```python
from build123d import *

# Parameters (mm, degrees)
HOLE1_D           = 16.0147
HOLE1_DEPTH       = 58.7248
HOLE1_CSINK_D     = 17.5387
HOLE1_CSINK_ANGLE = 90


with BuildPart() as part:
    # Sketch1 → Revolve1 (revolve)
    with BuildSketch(Plane.XY):
        with BuildLine():
            Line((0, 0), (0, 14.61516))
            Line((0, 14.61516), (1.25984, 15.875))
            Line((1.25984, 15.875), (12.006992339, 15.875))
            Line((12.006992339, 15.875), (13.283429147, 14.641164804))
            ThreePointArc((13.283429147, 14.641164804), (13.72258185, 14.355749006), (14.2367, 14.25575))
            Line((14.2367, 14.25575), (16.1036, 14.25575))
            ThreePointArc((16.1036, 14.25575), (17.073467661, 14.657482339), (17.4752, 15.62735))
            Line((17.4752, 15.62735), (17.4752, 17.44345))
            Line((17.4752, 17.44345), (20.6502, 17.44345))
            Line((20.6502, 17.44345), (20.6502, 0))
            Line((20.6502, 0), (0, 0))
        make_face()
    revolve(axis=Axis((20.6502, 0, 0), (-1, 0, 0)))

    # Sketch2 → Revolve2 (revolve)
    with BuildSketch(Plane.XY):
        Polygon((20.6502, 0), (20.6502, 24.96185), (22.1742, 26.48585), (49.1998, 26.48585), (49.1998, 24.51735), (50.2539, 24.51735), (51.308, 25.57145), (57.9628, 25.57145), (58.7248, 24.80945), (58.7248, 0), align=None)
    revolve(axis=Axis((58.7248, 0, 0), (-1, 0, 0)))

    # Hole1
    with Locations(Plane.ZY):
        with Locations((0, 0)):
            CounterSinkHole(HOLE1_D / 2, HOLE1_CSINK_D / 2, depth=HOLE1_DEPTH, counter_sink_angle=HOLE1_CSINK_ANGLE)

    # Sketch5 → Cut-Revolve1 (revolve, cut)
    with BuildSketch(Plane(origin=(0, 0, 0), x_dir=(1, 0, 0), z_dir=(0, 1, 0))):
        Polygon((39.1668, 0), (42.3418, 0), (42.3418, -8.986753545), (45.108896455, -11.75385), (45.568822746, -26.48585), (39.1668, -26.48585), align=None)
    revolve(axis=Axis((39.1668, 0, 26.48585), (0, 0, -1)), mode=Mode.SUBTRACT)

    # Sketch6 → Revolve3 (revolve)
    with BuildSketch(Plane.XY):
        with BuildLine():
            Line((49.1998, 24.26335), (50.2539, 24.26335))
            Line((50.2539, 24.26335), (50.2539, 24.51735))
            Line((50.2539, 24.51735), (49.72685, 24.51735))
            Line((49.72685, 24.51735), (49.334816303, 24.909383697))
            ThreePointArc((49.334816303, 24.909383697), (49.297618864, 24.999186258), (49.334816303, 25.088988819))
            Line((49.334816303, 25.088988819), (50.647509288, 26.401681804))
            Line((50.647509288, 26.401681804), (50.647509288, 26.48585))
            Line((50.647509288, 26.48585), (50.444309288, 26.48585))
            Line((50.444309288, 26.48585), (49.1998, 25.241340712))
            Line((49.1998, 25.241340712), (49.1998, 24.26335))
        make_face()
    revolve(axis=Axis((50.2539, 0, 0), (-1, 0, 0)))


solid = part.part
```
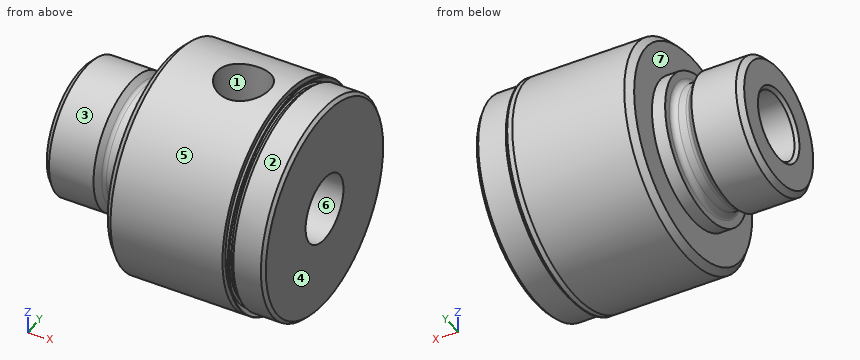
Here's how the part is built. I have some questions about the finished solid (model axes, mm). Face numbers are marked on the shaded views. A direction names the side the tool comes from. Coordinates: 2 decimals unless noted, no trailing zeros. Order: outer loops, then holes, each group sorted by start corner. A loop starts at its lowest first (then second) coordinate and runs counter-clockwise, first axis right, second up.
Item 1: Which directions (+Z, -Z, +X, -X, +Y, -Y) give clear straight access to the entire face, cutting with the end or side of a thin tool? Please do the marked faces 1, 2, 3 and 4.
Response values:
face 1: +Z
face 2: +X
face 3: -X
face 4: +Z, -Z, +X, +Y, -Y
Item 2: If we section it at A-A, the plane x = 8.5: List the corners of the cut face in (y, z) for me (3 decimals), then the cut area to 3 significant figures.
Response values:
outline: circle Ø31.75 at (0, 0); hole circle Ø16.015 at (0, 0)
area: 590 mm2
Item 3: If we section it at B-B, the plane y = 0: Give the number of separate pieces and of enclosed holes in the cut face, then the cut area to 3 significant figures.
Response values:
separate pieces: 3
enclosed holes: 0
area: 1,490 mm2
Item 4: Thinking about a two-plate mould opening in Y: for the marked faces 5, 6 and 7, which applies, pulls with the +Y half, pulls with the -Y half, needs draft (parallel to the pull), parting line crosses it, or undercut?
Response values:
face 5: parting line crosses it
face 6: undercut
face 7: needs draft
Item 5: I'm going to push flat-ended pins straight in: pin 1 Ø2 at (x, y) = (35, -18) entering from +Z; pin 2 Ø1 at (x, z) = (52.5, -5.5) entering from -Y; pin 3 Ø3 at (x, z) = (27.5, -7.5) entering from -Y. Where does each tip first touch, or does it pass through?
Response values:
pin 1: stops at z = 20.31
pin 2: stops at y = -25.08
pin 3: stops at y = -25.8
Item 6: I need wall thicknesses on probe 1 along Y at (x, z) = (42, 0); probe 2 along Y at (x, z) = (20, -0.5); probe 3 along Y at (x, z) = (50, 20). Which ranges of each line are inside material? Lowest first, please.
Response values:
probe 1: y = -26.49 to -8.01, 8.01 to 26.49
probe 2: y = -17.44 to -7.99, 7.99 to 17.44
probe 3: y = -16.68 to -16.23, -14.18 to 14.18, 16.23 to 16.68
